Input: part model. Units: mm. Frame: model coordinates. Coordinates: 2 decimals unless noted, no trailing zeros. Write each loop counter-clockwise with the first axis right and the second up, starting at its lowest first coordinate (ties: lowest second). Pieces come first, ordered by that corner, then holes. Notation, with made-up numbers: M 11,20 L 51,20 A9 cw 51,29 Z; hole C 50.25,-38 d7. An arc over 180 degrees is marked long. Use one line per item in the form item = value.
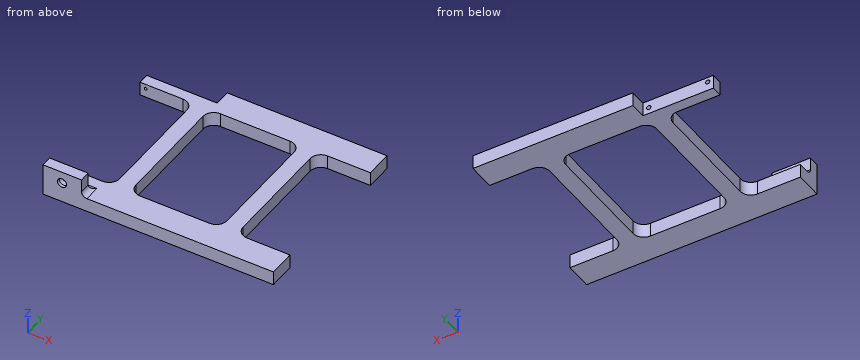
from build123d import *

# Parameters (mm, degrees)
F0_W      = 36
F0_H      = 10
F1_DEPTH  = 13
F3_R      = 2
F4_DEPTH  = 10
F4_TAPER  = 4
F5_DEPTH  = 30
F6_R      = 5
F8_R      = 4.25
F9_DEPTH  = 12.5
F8_R_2    = 4.5
F10_DEPTH = 2.25


# Not quite as in the source:
# - a feature names something its author has since deleted; it is built from what else it names


with BuildPart() as f1:
    # F0 (on Top) → F1 (new body)
    with BuildSketch(Plane.XY):
        with BuildLine():
            Line((-41.7, 85.5), (-41.7, 70.5))
            Line((-41.7, 70.5), (-107.5, 70.5))
            Line((-107.5, 70.5), (-107.5, 60.5))
            Line((-107.5, 60.5), (-67.5, 60.5))
            ThreePointArc((-67.5, 60.5), (-60.4289321881, 57.5710678119), (-57.5, 50.5))
            Line((-57.5, 50.5), (-57.5, -50.5))
            ThreePointArc((-57.5, -50.5), (-60.4289321881, -57.5710678119), (-67.5, -60.5))
            Line((-67.5, -60.5), (-107.5, -60.5))
            Line((-107.5, -60.5), (-107.5, -70.5))
            Line((-107.5, -70.5), (-107.5, -75.5))
            Line((-107.5, -75.5), (-71.5, -75.5))
            Line((-71.5, -75.5), (-71.5, -85.5))
            Line((-71.5, -85.5), (41.7, -85.5))
            Line((41.7, -85.5), (107.5, -85.5))
            Line((107.5, -85.5), (107.5, -70.5))
            Line((107.5, -70.5), (107.5, -60.5))
            Line((107.5, -60.5), (67.5, -60.5))
            ThreePointArc((67.5, -60.5), (60.4289321881, -57.5710678119), (57.5, -50.5))
            Line((57.5, -50.5), (57.5, 50.5))
            ThreePointArc((57.5, 50.5), (60.4289321881, 57.5710678119), (67.5, 60.5))
            Line((67.5, 60.5), (107.5, 60.5))
            Line((107.5, 60.5), (107.5, 70.5))
            Line((107.5, 70.5), (107.5, 85.5))
            Line((107.5, 85.5), (-41.7, 85.5))
        make_face()
        with BuildLine():
            Line((-32.5, 60.5), (32.5, 60.5))
            ThreePointArc((32.5, 60.5), (39.5710678119, 57.5710678119), (42.5, 50.5))
            Line((42.5, 50.5), (42.5, -50.5))
            ThreePointArc((42.5, -50.5), (39.5710678119, -57.5710678119), (32.5, -60.5))
            Line((32.5, -60.5), (-32.5, -60.5))
            ThreePointArc((-32.5, -60.5), (-39.5710678119, -57.5710678119), (-42.5, -50.5))
            Line((-42.5, -50.5), (-42.5, 50.5))
            ThreePointArc((-42.5, 50.5), (-39.5710678119, 57.5710678119), (-32.5, 60.5))
        make_face(mode=Mode.SUBTRACT)
        with Locations((-89.5, -80.5)):
            Rectangle(F0_W, F0_H)
    extrude(amount=F1_DEPTH)

    # F3 (on offset) → F4 (cut)
    with BuildSketch(Plane(origin=(0, 70.5, 0), x_dir=(-1, 0, 0), z_dir=(0, 1, 0))):
        with Locations((47.2, 6)):
            Circle(F3_R)
        with Locations((102.2, 8.5)):
            Circle(F3_R)
    extrude(amount=-F4_DEPTH, taper=F4_TAPER, mode=Mode.SUBTRACT)

    # F0 (on Top) → F5 (join)
    with BuildSketch(Plane.XY):
        with Locations((-89.5, -80.5)):
            Rectangle(F0_W, F0_H)
    extrude(amount=F5_DEPTH)

    # F6
    f6_edges = [f1.edges().sort_by_distance(p)[0] for p in [
        (-89.5, -75.5, 13),
        (-71.5, -80.5, 13),
    ]]
    fillet(f6_edges, radius=F6_R)

    # F8 (on offset) → F9 (cut, symmetric)
    with BuildSketch(Plane.XZ.offset(80.5)):
        with Locations((-89.8, 19)):
            Circle(F8_R)
    extrude(amount=F9_DEPTH, both=True, mode=Mode.SUBTRACT)

    # F8 (on offset) → F10 (cut, symmetric)
    with BuildSketch(Plane.XZ.offset(80.5)):
        with Locations((-89.8, 19)):
            Circle(F8_R_2)
        with Locations((-89.8, 19)):
            Circle(F8_R, mode=Mode.SUBTRACT)
    extrude(amount=F10_DEPTH, both=True, mode=Mode.SUBTRACT)


solid = f1.part
(1) Line query: probe 1 along Y at (x, z) = (-3.5, 9); probe 2 along X at (y, z) = (34, 5); probe 3 along X at (y, z) = (-77.1, 19). Output: solid intervals per line, ascending.
Computed:
probe_1 = -85.5 to -60.5, 60.5 to 85.5
probe_2 = -57.5 to -42.5, 42.5 to 57.5
probe_3 = -107.5 to -94.05, -85.55 to -71.5
(2) First-contact query: pin 1 Ø14.5 at (y, z) = (1.5, 5.5) entering from -X; pin 2 Ø3.5 at (x, z) = (-88, 26) entering from +Y; pin 3 Ø4 at (x, z) = (-92.5, 6.5) entering from +Y; pin 4 Ø8 at (x, y) = (37, -36.5) entering from -Z. Flat tips, straight axial feed; report the tip coordinate or a pass-through.
Computed:
pin_1 = -57.5
pin_2 = -75.5
pin_3 = 70.5
pin_4 = through
(3) Section query C-C on x = -89.8. Return the cut outline in (y, z), plus the area to 3 significant figures.
Computed:
outline = M -85.5,0 L -60.5,0 L -60.5,13 L -70.5,13 A5 cw -74.3,14.75 L -78.25,14.75 L -78.25,14.5 L -82.75,14.5 L -82.75,14.75 L -85.5,14.75 Z; M -85.5,23.25 L -82.75,23.25 L -82.75,23.5 L -78.25,23.5 L -78.25,23.25 L -75.5,23.25 L -75.5,30 L -85.5,30 Z; M 60.5,0 L 70.5,0 L 70.5,13 L 60.5,13 Z
area = 542 mm^2
(4) Section query B-B on x = 80. Return the cut outline in (y, z), plus the area to 3 significant figures.
Computed:
outline = M -85.5,0 L -60.5,0 L -60.5,13 L -85.5,13 Z; M 60.5,0 L 85.5,0 L 85.5,13 L 60.5,13 Z
area = 650 mm^2
(5) Section query A-A on y = 4.5. Return the cut outline in (x, z), plus the area to 3 significant figures.
Computed:
outline = M -57.5,0 L -42.5,0 L -42.5,13 L -57.5,13 Z; M 42.5,0 L 57.5,0 L 57.5,13 L 42.5,13 Z
area = 390 mm^2
